CAD build for the part. Positions are in the model's coordinates, mm. Round coordinates to 2 decimals unless told otherwise and drop trailing zeros. Loops run counter-clockwise (first coordinate to the right, second up) from the corner with the lowest first, then second, coordinate; pieces in that order, holes last. Notation, with made-up numbers: M -16,0 L -7,0 A20 ccw -7,20 Z; hole C 46,87 d5. An arc over 180 degrees is marked long. One line per item, written item: value. Start each with the question number.
from build123d import *

# Parameters (mm, degrees)
SKETCH1_R           = 1.4
BOSS_EXTRUDE1_DEPTH = 3.175
FILLET1_R           = 10
FILLET2_R           = 3


with BuildPart() as part:
    # Sketch1 → Boss-Extrude1 (new body)
    with BuildSketch(Plane.XY):
        Polygon((9, 9), (9, 81), (0, 81), (0, -32), (52, -32), (52, 9), align=None)
        with Locations((4.5, 5.5)):
            Circle(SKETCH1_R, mode=Mode.SUBTRACT)
        with Locations((4.5, 74.47)):
            Circle(SKETCH1_R, mode=Mode.SUBTRACT)
    extrude(amount=BOSS_EXTRUDE1_DEPTH)

    # Fillet1
    fillet1_edges = [part.edges().sort_by_distance(p)[0] for p in [
        (9, 9, 1.5875),
    ]]
    fillet(fillet1_edges, radius=FILLET1_R)

    # Fillet2
    fillet2_edges = [part.edges().sort_by_distance(p)[0] for p in [
        (9, 81, 1.5875),
        (52, 9, 1.5875),
    ]]
    fillet(fillet2_edges, radius=FILLET2_R)


solid = part.part
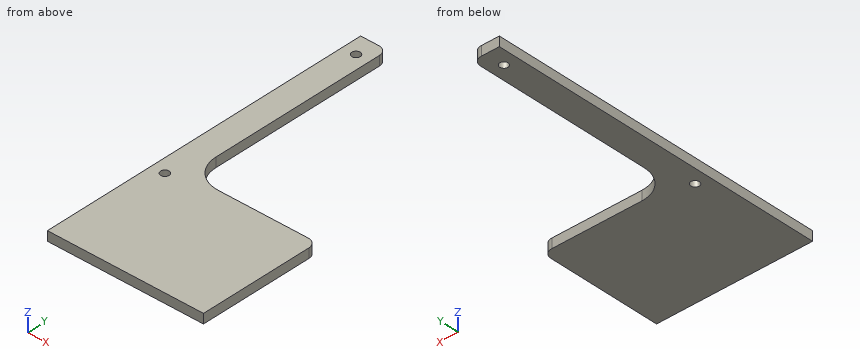
(1) Probe L1, parallel to Y at x = 4.5, z = 2.2; L2, parallel to X at y = 42, z = 1.95; L3, parallel to Y at x = 47, z = 1.15. List the from-to ranges inside material, lowest first.
(2) Flat gauge pins, fed straight in: P1, Ø2, axis at x = 4.5, y = 5.5, coming from the -Z side; P2, Ø1.5, axis at y = 31, z = 2, coming from the +X side; P3, Ø4.5, axis at x = 4.5, y = 74.47, coming from the -Z side. Where does each tip first touch, or does it go through?
(3) Slice it at D-D, the plane y = 37. List the corners of the cut face in (x, z) (3 decimals), and give its area (3 significant figures).
(4) Slice it at B-B, the plane z = 0.65. List the corners of the cut face in (x, y).
(5) Slice it at A-A, the plane y = 74.47. List the corners of the cut face in (x, z) (3 decimals), and give its area (3 significant figures).
(6) Slice it at C-C, the plane x = 47.5. List the corners of the cut face in (y, z) (3 decimals), and give its area (3 significant figures).
Check result:
1. L1: y = -32 to 4.1, 6.9 to 73.07, 75.87 to 81
1. L2: x = 0 to 9
1. L3: y = -32 to 9
2. P1: passes through
2. P2: stops at x = 9
2. P3: stops at z = 0
3. outline: M 0,0 L 9,0 L 9,3.175 L 0,3.175 Z
3. area: 28.6 mm^2
4. outline: M 0,-32 L 52,-32 L 52,6 A3 ccw 49,9 L 19,9 A10 cw 9,19 L 9,78 A3 ccw 6,81 L 0,81 Z; hole C 4.5,5.5 d2.8; hole C 4.5,74.47 d2.8
5. outline: M 0,0 L 3.1,0 L 3.1,3.175 L 0,3.175 Z; M 5.9,0 L 9,0 L 9,3.175 L 5.9,3.175 Z
5. area: 19.7 mm^2
6. outline: M -32,0 L 9,0 L 9,3.175 L -32,3.175 Z
6. area: 130 mm^2
